Verification items for this drawing (mm, ordinates from the low corner). A direction names the side the tool comes from. Give positions to 0.01 mm unless a question says otherwise; leave off trailing zeros. Order: outer loops, then holes, each group sorted by start corner. A loop starts at its lowest first (then second) coordinate and runs counter-clockwise, first axis right, second up. Notation, with made-up numbers: (27, -34) - (77, -34) arc R25 cw to (77, 4) - close; hole circle Ø11 at (-4, 16). An arc over 180 degrees is marked (long way). Put each result on its own line as item: value. Start each with the question number.
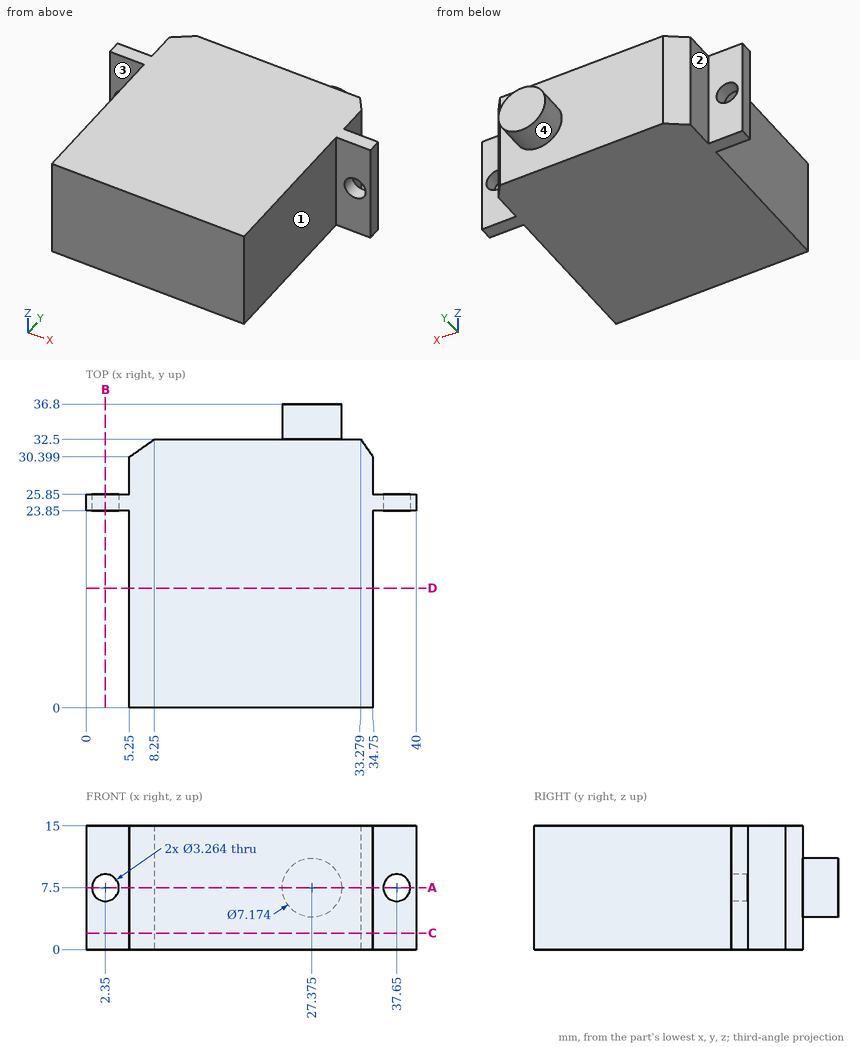
Item 1: Cross-section at B-B (x = 2.35). Enter the section's corners in (y, z).
Item 2: Thickness scan on line 1 along X through (y, z) = (25.4, 7.5); line 2 along Z through (x, y) = (37.65, 24.75); line 3 along Y through (x, z) = (10, 4.5). Record the ranges inside material, lowest first.
Item 3: Cross-section at D-D (y = 14.5). Enter the section's corners in (x, z).
Item 4: Set-up check for the marked faces 1, 2, 3 and 4: record each of +Z, -Z, +X, -X, +Y, -Y from which the full face is reachable in a straight line by a thin tool's end or side.
Item 5: Gauge pin test, flat ends, axial feed: pin 1 Ø6 at (x, z) = (38.5, 5) entering from -Y; pin 2 Ø7.5 at (y, z) = (17.5, 10) entering from +X; pin 3 Ø2.5 at (x, z) = (1.5, 6) entering from +Y. Record the tip position at first contact, or that the pin passes through.
Item 6: Cross-section at A-A (z = 7.5). Enter the section's corners in (x, y), and give its area (3 significant figures).
Item 7: Cross-section at C-C (z = 2). Enter the section's corners in (x, y).
Recorded:
1. outline: (23.85, 0) - (25.85, 0) - (25.85, 5.87) - (23.85, 5.87) - close; (23.85, 9.13) - (25.85, 9.13) - (25.85, 15) - (23.85, 15) - close
2. line 1: x = 0 to 0.72, 3.98 to 36.02, 39.28 to 40
2. line 2: z = 0 to 5.87, 9.13 to 15
2. line 3: y = 0 to 32.5
3. outline: (5.25, 0) - (34.75, 0) - (34.75, 15) - (5.25, 15) - close
4. face 1: +Z, -Z, +X, -Y
4. face 2: +Z, -Z, -X, +Y
4. face 3: +Z, -Z, -X, -Y
4. face 4: +Y
5. pin 1: stops at y = 23.85
5. pin 2: stops at x = 34.75
5. pin 3: stops at y = 25.85
6. outline: (0, 23.85) - (0.72, 23.85) - (0.72, 25.85) - (0, 25.85) - close; (3.98, 23.85) - (5.25, 23.85) - (5.25, 0) - (34.75, 0) - (34.75, 23.85) - (36.02, 23.85) - (36.02, 25.85) - (34.75, 25.85) - (34.75, 30.4) - (33.28, 32.5) - (30.96, 32.5) - (30.96, 36.8) - (23.79, 36.8) - (23.79, 32.5) - (8.25, 32.5) - (5.25, 30.4) - (5.25, 25.85) - (3.98, 25.85) - close; (39.28, 23.85) - (40, 23.85) - (40, 25.85) - (39.28, 25.85) - close
6. area: 993 mm^2
7. outline: (0, 23.85) - (5.25, 23.85) - (5.25, 0) - (34.75, 0) - (34.75, 23.85) - (40, 23.85) - (40, 25.85) - (34.75, 25.85) - (34.75, 30.4) - (33.28, 32.5) - (8.25, 32.5) - (5.25, 30.4) - (5.25, 25.85) - (0, 25.85) - close
